The listing builds one solid part. Answer for the finished solid, in the listing's coordinates (mm). Coordinates: 2 decimals unless noted, no trailing zeros. Order: outer loops, then holes, each group sorted by start corner. A loop starts at its lowest first (then second) coordinate and runs counter-clockwise, first axis right, second up. Notation, with made-up numbers: (51.5, -35) - (97.5, -35) arc R4 cw to (97.5, -29) - close; hole circle Ø11 at (4.5, 15). An arc over 180 degrees is marked (long way). Use a Markdown table: item, result. Add a question column.
Item 1: The mould has two halves that part along Y. Classify faces 1 (the cylindrical face through (-18.73, -10.89, 2.35)), 2 (the cylindrical face through (-18.827, 10.79, 2.348)), 3 (the cylindrical face through (-13.854, 2.545, 2.348)): released by +Y, released by -Y, zero draft, split by the parting line, or undercut.
Item 2: The part is cut by section A-A, the plane x = 12.7. Give the vertices of the cut face in (y, z), then the cut area to 3 significant figures.
Item 3: The part is cut by section B-B, the plane z = 2.8. Give the vertices of the cut face in (x, y).
Item 4: Flat-ended cylindrical pins translate along their axes: P1, Ø4.5, axis at x = -12.7, y = 4.76, coming from the +Z side; P2, Ø1, axis at y = 9.5, z = 3.5, coming from the -X side. Find the tip coordinate at first contact, or state that the pin passes through.
Item 5: The part is cut by section D-D, the plane x = -13. Give the vertices of the cut face in (y, z), then the cut area to 3 significant figures.
Item 6: The part is cut by section C-C, the plane y = 5.75. Give the vertices of the cut face in (x, z).
Item 7: Find the intervals of material crossed by line 1 along X through (y, z) = (6.5, 2.5); line 2 along Y through (x, z) = (-12.7, 2); line 3 along X through (y, z) = (3.75, 0.55), in increasing order.
from build123d import *

# Parameters (mm, degrees)
SKETCH1_W             = 41.275
SKETCH1_H             = 25.4
BASE_FLANGE1_DEPTH    = 4.7625
BREAK_CORNER1_DEPTH   = 4.7625
M6X1_0_TAPPED_HOLE1_D = 5


# Read off the part's stored shape, not the designer's step: Break-Corner1
# Sheet-metal steps are written as plain solids
with BuildPart() as part:
    # Sketch1 → Base-Flange1 (new body)
    with BuildSketch(Plane.XY):
        Rectangle(SKETCH1_W, SKETCH1_H)
    extrude(amount=BASE_FLANGE1_DEPTH)

    # Break-Corner1 outline → Break-Corner1 (cut)
    with BuildSketch(Plane.XY):
        with BuildLine():
            Line((-20.6375, 12.7), (-20.6375, 6.35))
            ThreePointArc((-20.6375, 6.35), (-18.777628061, 10.840128061), (-14.2875, 12.7))
            Line((-14.2875, 12.7), (-20.6375, 12.7))
        make_face()
        with BuildLine():
            ThreePointArc((-14.2875, -12.7), (-18.777628061, -10.840128061), (-20.6375, -6.35))
            Line((-20.6375, -6.35), (-20.6375, -12.7))
            Line((-20.6375, -12.7), (-14.2875, -12.7))
        make_face()
        with BuildLine():
            Line((20.6375, 12.7), (14.2875, 12.7))
            ThreePointArc((14.2875, 12.7), (18.777628061, 10.840128061), (20.6375, 6.35))
            Line((20.6375, 6.35), (20.6375, 12.7))
        make_face()
        with BuildLine():
            ThreePointArc((20.6375, -6.35), (18.777628061, -10.840128061), (14.2875, -12.7))
            Line((14.2875, -12.7), (20.6375, -12.7))
            Line((20.6375, -12.7), (20.6375, -6.35))
        make_face()
    extrude(amount=BREAK_CORNER1_DEPTH, mode=Mode.SUBTRACT)

    # M6x1.0 Tapped Hole1 (through all)
    with Locations(Plane.XY.offset(4.7625)):
        with Locations((-12.7, 4.7625), (12.7, 4.7625)):
            Hole(M6X1_0_TAPPED_HOLE1_D / 2)


solid = part.part
Solution:
| question | item | result |
|---|---|---|
| 1 | face 1 | released by -Y |
| 1 | face 2 | released by +Y |
| 1 | face 3 | undercut |
| 2 | outline | (-12.7, 0) - (2.26, 0) - (2.26, 4.76) - (-12.7, 4.76) - close; (7.26, 0) - (12.7, 0) - (12.7, 4.76) - (7.26, 4.76) - close |
| 2 | area | 97.2 mm2 |
| 3 | outline | (-20.64, -6.35) arc R6.35 ccw to (-14.29, -12.7) - (14.29, -12.7) arc R6.35 ccw to (20.64, -6.35) - (20.64, 6.35) arc R6.35 ccw to (14.29, 12.7) - (-14.29, 12.7) arc R6.35 ccw to (-20.64, 6.35) - close; hole circle Ø5 at (-12.7, 4.76); hole circle Ø5 at (12.7, 4.76) |
| 4 | P1 | passes through |
| 4 | P2 | stops at x = -20.06 |
| 5 | outline | (-12.7, 0) - (2.28, 0) - (2.28, 4.76) - (-12.7, 4.76) - close; (7.24, 0) - (12.7, 0) - (12.7, 4.76) - (7.24, 4.76) - close |
| 5 | area | 97.3 mm2 |
| 6 | outline | (-20.64, 0) - (-15, 0) - (-15, 4.76) - (-20.64, 4.76) - close; (-10.4, 0) - (10.4, 0) - (10.4, 4.76) - (-10.4, 4.76) - close; (15, 0) - (20.64, 0) - (20.64, 4.76) - (15, 4.76) - close |
| 7 | line 1 | x = -20.64 to -14.5, -10.9 to 10.9, 14.5 to 20.64 |
| 7 | line 2 | y = -12.7 to 2.26, 7.26 to 12.7 |
| 7 | line 3 | x = -20.64 to -14.99, -10.41 to 10.41, 14.99 to 20.64 |
